Verification items for the finished model (mm, model axes). Face numbers are marked on the shaded views. A direction names the side the tool comes from. Give positions to 0.01 mm unless a question says otherwise; leave off trailing zeros. Write each loop counter-clockwise with the first axis right and the second up, starting at its lowest first coordinate (ties: lowest second). Pieces come first, ordered by that corner, then holes. Notation, with made-up numbers: (5.25, 80.5) - (39.25, 80.5) arc R12 ccw to (39.25, 98.5) - close; hole circle Ø9 at (59, -32.75). An arc over 180 degrees is marked (long way). Answer as a JSON object with one key per item and string values. Group by question number.
Item 1: Tool access check on the marked faces 4 and 5. Record the directions out of +Z, -Z, +X, -X, +Y, -Y that give a thin tool (end or side, any length) a straight path to the whole face; none if there is none.
Item 2: Sectioned sample at D-D, the plane x = 39.5. Record the boundary of the cut face in (y, z).
Item 3: Sectioned sample at A-A, the plane x = -25.4. Record the boundary of the cut face in (y, z), and give its area (3 significant figures).
Item 4: Draft check along X on the marked faces 1, 2 and 3. Enter one of: +X half, -X half, draft (parallel to the pull), parting line (faces both ways), or undercut.
Item 5: Sectioned sample at C-C, the plane z = 34.5. Record the boundary of the cut face in (x, y), and give its area (3 significant figures).
Item 6: Go/stop test with flat-tipped pins: pin 1 (3 mm diameter, centred on x = 60, z = 2, fed in from -Y); pin 2 (20.5 mm diameter, centred on x = 58.5, y = 66, fed in from +Z); pin 3 (7.5 mm diameter, centred on y = 59, z = 38, fed in from +X); pin 4 (4 mm diameter, centred on x = 61, y = 59.5, fed in from +Z). Record where each tip stops, or that it passes through.
Item 7: Scan lines: line 1 along Z through (x, y) = (-25, 55); line 2 along X through (y, z) = (44.5, 0); line 3 along Z through (x, y) = (69, 54.5). Record each from-to range of solid material in increasing order. Write a range as [from, to].
Item 8: Sectioned sample at B-B, the plane y = 53. Record the boundary of the cut face in (x, z), and give its area (3 significant figures).
```python
from build123d import *

# Parameters (mm, degrees)
SKETCH1_W           = 152.4
SKETCH1_H           = 101.6
BOSS_EXTRUDE1_DEPTH = 76.2
CUT_EXTRUDE1_DEPTH  = 25.4
SKETCH3_R           = 23.033719166
CUT_EXTRUDE2_DEPTH  = 120.1365603


with BuildPart() as part:
    # Sketch1 → Boss-Extrude1 (new body)
    with BuildSketch(Plane(origin=(0, 0, 0), x_dir=(1, 0, 0), z_dir=(0, 1, 0))):
        Rectangle(SKETCH1_W, SKETCH1_H)
    extrude(amount=BOSS_EXTRUDE1_DEPTH)

    # Sketch2 → Cut-Extrude1 (cut)
    with BuildSketch(Plane(origin=(0, 76.2, 0), x_dir=(1, 0, 0), z_dir=(0, 1, 0))):
        Polygon((76.2, -50.8), (25.4, -50.8), (25.4, 0), (50.8, 0), (50.8, 25.4), (76.2, 25.4), (76.2, 15.210104037), align=None)
    extrude(amount=-CUT_EXTRUDE1_DEPTH, mode=Mode.SUBTRACT)

    # Sketch3 → Cut-Extrude2 (cut, through all)
    with BuildSketch(Plane(origin=(0, 76.2, 0), x_dir=(1, 0, 0), z_dir=(0, 1, 0))):
        with Locations(Location((-25.4, 0, 0), (0, 0, 270))):
            Circle(SKETCH3_R)
    extrude(amount=-CUT_EXTRUDE2_DEPTH, mode=Mode.SUBTRACT)


solid = part.part
```
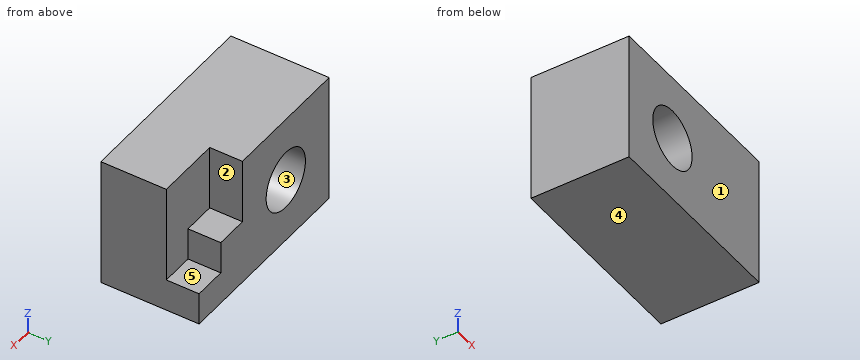
Geometry check:
{
 "1": {"face 4": "-Z, +X, -X, +Y, -Y", "face 5": "+Z, +X, +Y"},
 "2": {"outline": "(0, -50.8) - (76.2, -50.8) - (76.2, 0) - (50.8, 0) - (50.8, 50.8) - (0, 50.8) - close"},
 "3": {"outline": "(0, -50.8) - (76.2, -50.8) - (76.2, -23.03) - (0, -23.03) - close; (0, 23.03) - (76.2, 23.03) - (76.2, 50.8) - (0, 50.8) - close", "area": "4,230 mm^2"},
 "4": {"face 1": "draft", "face 2": "+X half", "face 3": "undercut"},
 "5": {"outline": "(-76.2, 0) - (76.2, 0) - (76.2, 50.8) - (25.4, 50.8) - (25.4, 76.2) - (-76.2, 76.2) - close", "area": "10,300 mm^2"},
 "6": {"pin 1": "y = 0", "pin 2": "z = 0", "pin 3": "x = 25.4", "pin 4": "z = -25.4"},
 "7": {"line 1": "[-50.8, -23.03], [23.03, 50.8]", "line 2": "[-76.2, -48.43], [-2.37, 76.2]", "line 3": "[-50.8, -25.4]"},
 "8": {"outline": "(-76.2, -50.8) - (76.2, -50.8) - (76.2, -25.4) - (50.8, -25.4) - (50.8, 0) - (25.4, 0) - (25.4, 50.8) - (-76.2, 50.8) - close; hole circle Ø46.07 at (-25.4, 0)", "area": "10,600 mm^2"}
}
